Geometry check sheet. Reference: drawing and pictorial views, mm from the part's lowest x, y, z. A direction names the side the tool comes from. Round coordinates to 2 decimals unless told otherwise and drop trailing zeros. Order: outer loops, then holes, each group sorted by start corner. A loop starts at its lowest first (then second) coordinate and runs counter-clockwise, first axis right, second up.
(1) Sectioned sample at B-B (x = 25.5). Record the boundary of the cut face in (y, z), plus the area to 4 significant figures.
(2) Sectioned sample at D-D (z = 65.5). Record the boundary of the cut face in (x, y), plus the area to 3 significant figures.
(3) Set-up check for the marked faces 4, 5, 6, 7 and 8: record each of +Z, -Z, +X, -X, +Y, -Y from which the full face is reachable in a straight line by a thin tool's end or side.
(4) Material ranges on line 1 along Z through (x, y) = (47.5, 5.5); line 2 along X through (y, z) = (4, 4); line 3 along Y through (x, z) = (37.5, 34), recorded low to high.
(5) Go/stop test with flat-tipped pins: pin 1 (12 mm diameter, centred on x = 30.5, z = 36, fed in from +Y); pin 2 (2.5 mm diameter, centred on y = 4, z = 15.5, fed in from -X); pin 3 (2 mm diameter, centred on x = 24, z = 46, fed in from +Y); pin 4 (25 mm diameter, centred on y = 37, z = 49, fed in from -X). Record where each tip stops, or that it passes through.
(6) Sectioned sample at A-A (y = 36). Record the boundary of the cut face in (x, z), plus the area to 3 significant figures.
(7) Release check for a two-part mould opening along Z. For the marked faces 1, 2 and 3 record: +Z half, -Z half, draft (parallel to the pull), parting line (faces both ways), or undercut.
(8) Sectioned sample at C-C (z = 7). Record the boundary of the cut face in (x, y).
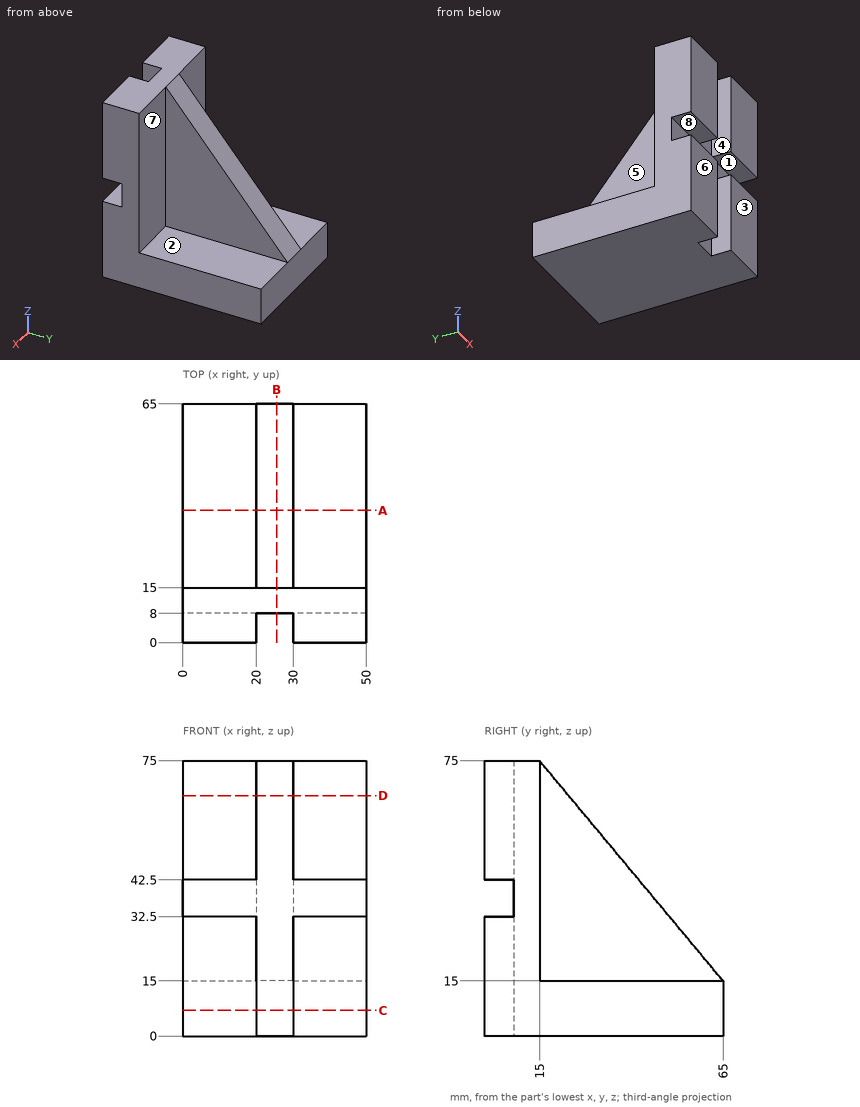
Answer below:
1. outline: (8, 0) - (65, 0) - (65, 15) - (15, 75) - (8, 75) - close
1. area: 2,775 mm2
2. outline: (0, 0) - (20, 0) - (20, 8) - (30, 8) - (30, 0) - (50, 0) - (50, 15) - (30, 15) - (30, 22.92) - (20, 22.92) - (20, 15) - (0, 15) - close
2. area: 749 mm2
3. face 4: +Z, -Z, -Y
3. face 5: +Z, -X, +Y
3. face 6: +Z, -Z, +X, -X, -Y
3. face 7: +Z, +X, +Y
3. face 8: +X, -X, -Y
4. line 1: z = 0 to 32.5, 42.5 to 75
4. line 2: x = 0 to 20, 30 to 50
4. line 3: y = 8 to 15
5. pin 1: stops at y = 52.48
5. pin 2: stops at x = 0
5. pin 3: stops at y = 40
5. pin 4: stops at x = 20
6. outline: (0, 0) - (50, 0) - (50, 15) - (30, 15) - (30, 49.8) - (20, 49.8) - (20, 15) - (0, 15) - close
6. area: 1,100 mm2
7. face 1: undercut
7. face 2: +Z half
7. face 3: draft
8. outline: (0, 0) - (20, 0) - (20, 8) - (30, 8) - (30, 0) - (50, 0) - (50, 65) - (0, 65) - close
